Autodesk Inventor part; units mm, degrees
ref_plane "Arbeitsebene1" through (60, 0, 0) normal (1, 0, 0) x (0, 1, 0)
ref_plane "Arbeitsebene2" through (0, 16, 0) normal (0, 1, 0) x (-1, 0, 0)
ref_plane "Arbeitsebene3" through (30, 0, 0) normal (1, 0, 0) x (0, 1, 0)
sketch "Skizze1" plane through (0, 0, 0) normal (0, 0, 1) x (1, 0, 0)
  line L0 (0, 0) -> (112, 0)
  line L1 (112, 0) -> (112, 28)
  line L2 (112, 28) -> (0, 28)
  line L3 (0, 28) -> (0, 0)
  dimension "d0" = 28
  dimension "d1" = 112
extrude "Extrusion1" add sketch "Skizze1" along normal blind 60
sketch "Skizze2" plane through (112, 0, 0) normal (1, 0, 0) x (0, 0, -1)
  line L0 (0, 0) -> (-60, 0)
  line L1 (-50, 0) -> (-50, 14)
  line L2 (-50, 14) -> (-10, 14)
  line L3 (-10, 14) -> (-10, 0)
  line L4 (-60, 0) -> (-60, 28)
  line L5 (0, 28) -> (-60, 28)
  point P0 (-10, 7)
  point P1 (-50, 7)
  point P2 (-30, 14)
  dimension "d4" = 40
  dimension "d5" = 10
  dimension "d6" = 14
extrude "Extrusion2" cut sketch "Skizze2" against normal up to surface (112 mm away)
sketch "Skizze3" plane through (0, 28, 0) normal (0, 1, 0) x (1, 0, 0)
  line L0 (112, -60) -> (0, -60)
  line L1 (0, 0) -> (112, 0)
  line L2 (0, -60) -> (52, -60)
  line L3 (52, -60) -> (52, 0)
  line L4 (52, 0) -> (0, 0)
  line L5 (0, 0) -> (0, -60)
  line L6 (112, 0) -> (112, -60)
  point P0 (52, -30)
  dimension "d9" = 60
extrude "Extrusion3" add sketch "Skizze3" along normal blind 60 contours L0 L5 L1 L3
ref_plane "Arbeitsebene1" through (60, 0, 0) normal (1, 0, 0) x (0, 1, 0)
sketch "Skizze7" plane through (60, 0, 0) normal (1, 0, 0) x (0, 1, 0)
  circle A0 centre (88, 30) radius 30
  circle A1 centre (88, 30) radius 16
  line L0 (28, 0) -> (28, 60)
  point P0 (0, 0)
  point P1 (28, 30)
  point P2 (28, 30)
  dimension "d25" = 60
  dimension "d26" = 32
  dimension "d27" = 60
extrude "Extrusion6" add sketch "Skizze7" against normal blind 68
extrude "Extrusion7" cut sketch "Skizze7" against normal blind 68 contours A1
ref_plane "Arbeitsebene2" through (0, 16, 0) normal (0, 1, 0) x (-1, 0, 0)
sketch "Skizze11" plane through (0, 16, 0) normal (0, 1, 0) x (-1, 0, 0)
  circle A0 centre (-27, 110) radius 15
  circle A1 centre (-27, 110) radius 8
  line L0 (-12, 110) -> (-12, 59.6136)
  line L1 (-42, 110) -> (-42, 59.6136)
  line L2 (-52, 60) -> (-52, 14)
  line L3 (0, 60) -> (-52, 60)
  point P0 (0, 0)
  point P1 (-52, 54)
  point P2 (-42, 60)
  point P3 (-12, 60)
  dimension "d42" = 30
  dimension "d43" = 16
  dimension "d44" = 10
  dimension "d45" = 50
extrude "Extrusion10" add sketch "Skizze11" along normal blind 24 contours A0
extrude "Extrusion11" add sketch "Skizze11" along normal blind 12 contours L0 L3 L1 A0
ref_plane "Arbeitsebene3" through (30, 0, 0) normal (1, 0, 0) x (0, 1, 0)
sketch "Skizze13" plane through (30, 0, 0) normal (1, 0, 0) x (0, 1, 0)
  line L0 (28, 95) -> (28, 110)
  line L1 (31, 56.123) -> (103, 56.123)
  line L2 (103, 56.123) -> (37, 95)
  line L3 (37, 95) -> (28, 95)
  line L4 (28, 95) -> (28, 56.123)
  line L5 (31, 56.123) -> (28, 56.123)
  line L6 (16, 110) -> (28, 110)
  line L7 (16, 110) -> (16, 110)
  line L8 (16, 110) -> (28, 110)
  line L9 (28, 110) -> (28, 110)
  line L10 (40, 95) -> (40, 125)
  line L11 (28, 95) -> (40, 95)
  point P0 (0, 0)
  point P1 (34, 95)
  dimension "d55" = 30.5
  dimension "d56" = 66
  dimension "d57" = 72
  dimension "d58" = 3
extrude "Extrusion12" add sketch "Skizze13" against normal blind 8
properties part number "Gary" material "Stahl, galvanisiert"
The listing builds one solid part. Answer for the finished solid, in the listing's coordinates (mm). A direction names the side the tool comes from. Round coordinates to 2 decimals unless told otherwise and drop trailing zeros. Order: outer loops, then holes, each group sorted by start corner. A loop starts at its lowest first (then second) coordinate and runs counter-clockwise, first axis right, second up. Notation, with made-up numbers: (-31.5, 77) -> (5.5, 77) arc R30 cw to (5.5, 111) -> close; hole circle Ø4 at (-30.75, 51). An arc over 180 degrees is marked (long way). Write each question's results on one line, items separated by ' | '. Start each with the question number.
Q1. Each of these flat-tipped pins is pushed along its axis until it touches: pin 1 (6 mm diameter, centred on x = 65, z = 27.5, fed in from +Y); pin 2 (19.5 mm diameter, centred on y = 67, z = 81.5, fed in from +X); pin 3 (9.5 mm diameter, centred on y = 21, z = 94.5, fed in from +X); pin 4 (6.5 mm diameter, centred on x = 26, y = 31.5, fed in from +Z). Where does it stop, or does it pass through?
Q2. Find section D-D (x = 83). Determine the outline of the cut face in (y, z), then the cut area to 3 significant figures.
Q3. Find section C-C (y = 21.5). Determine the outline of the cut face in (x, z).
Q4. Find section B-B (z = 30). Determine the outline of the cut face in (x, y).
Q5. Find section A-A (y = 33.5). Determine the outline of the cut face in (x, z).
Q6. Which of the six approach directions +Z, -Z, +X, -X, +Y, -Y give full straight-line access (tool end or side, diameter ignored) to faces 1 (the flat face through (30, 48, 72)), 2 (the flat face through (60, 101, 17)), 3 (the cylindrical face through (26.476, 75.303, 20.264)), 4 (the flat face through (57, 7, 50))?
Q7. The mould has two halves that part along X. Classify faces 5 (the flat face through (112, 17, 30)), 6 (the cylindrical face through (28.73, 27.83, 117.81)), 7 (the flat face through (57, 7, 10)), 8 (the flat face through (12, 22, 85)): pulls with the +X half, pulls with the -X half, needs draft (parallel to the pull), parting line crosses it, or undercut.
Q8. Straight lines are drawn through the part: probe 1 along Z at (x, y) = (45, 88); probe 2 along Z at (x, y) = (27, 22); probe 3 along X at (y, z) = (61, 78). For each, find the intervals that lie inside material, in ascending order. Write a range as from..to.
Worked answers:
1) pin 1: stops at y = 28 | pin 2: stops at x = 30 | pin 3: stops at x = 42 | pin 4: stops at z = 125
2) outline: (0, 0) -> (28, 0) -> (28, 60) -> (0, 60) -> (0, 50) -> (14, 50) -> (14, 10) -> (0, 10) -> close | area: 1,120 mm2
3) outline: (0, 0) -> (112, 0) -> (112, 60) -> (42, 60) -> (42, 110) arc R15 ccw to (12, 110) -> (12, 60) -> (0, 60) -> close; hole circle Ø16 at (27, 110)
4) outline: (-8, 58) -> (0, 58) -> (0, 14) -> (112, 14) -> (112, 28) -> (52, 28) -> (52, 58) -> (60, 58) -> (60, 72) -> (-8, 72) -> close; (-8, 104) -> (60, 104) -> (60, 118) -> (-8, 118) -> close
5) outline: (0, 0) -> (52, 0) -> (52, 60) -> (30, 60) -> (30, 95) -> (22, 95) -> (22, 60) -> (0, 60) -> close; circle Ø30 at (27, 110); hole circle Ø16 at (27, 110)
6) face 1: +X, +Y | face 2: +Z, -Z, +X, +Y | face 3: +X, -X | face 4: +X, -X, -Y
7) face 5: pulls with the +X half | face 6: undercut | face 7: needs draft | face 8: pulls with the -X half
8) probe 1: z = 0..14, 46..60 | probe 2: z = 0..102, 118..125 | probe 3: x = 22..30
